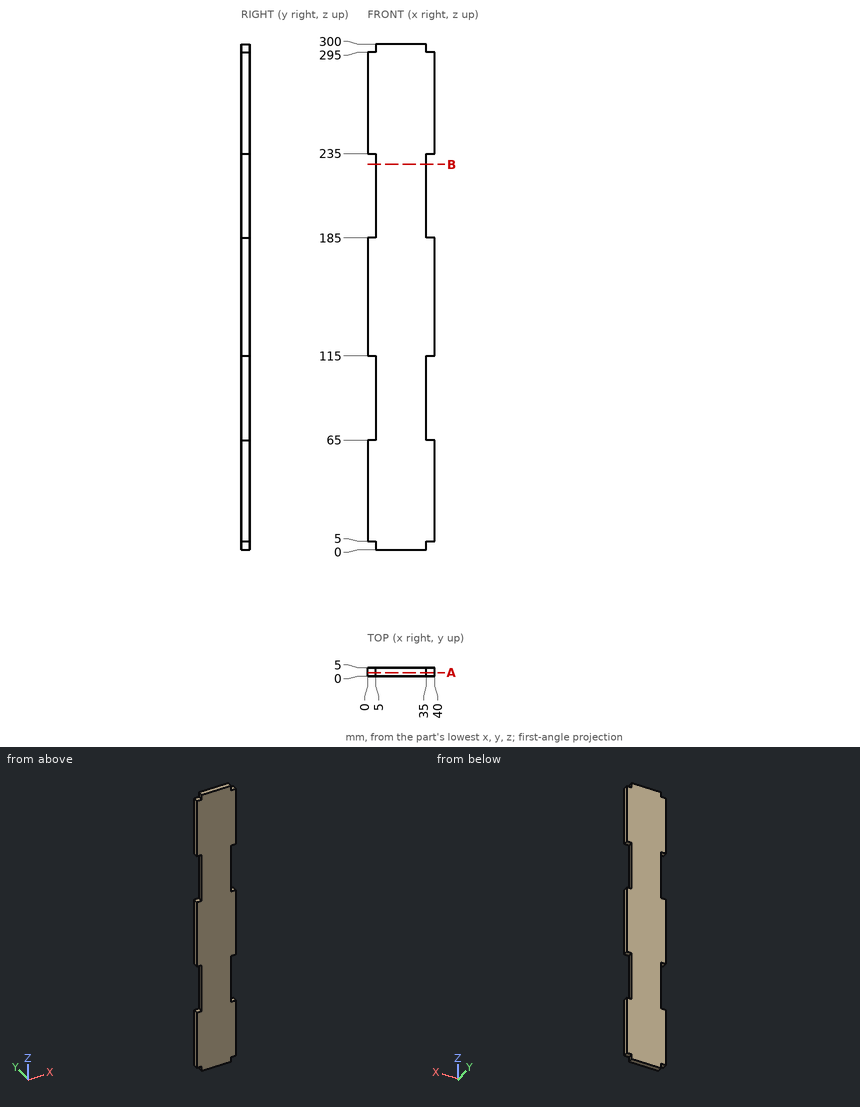
Answer from the drawing. Dimensions are ordinates in mm from the lowest x, y and z of the part. Round coordinates to 2 decimals unless told otherwise and drop trailing zeros. Order: outer loops, then holes, each group sorted by start corner. A loop starts at its lowest first (then second) coordinate and runs counter-clockwise, first axis right, second up.
1) The part is cut by section A-A on y = 2. Write down the section's boundary in (x, z).
2) Straight lines are drawn through the part: L1, parallel to Z at x = 3.5, y = 3.95; L2, parallel to X at y = 0.75, z = 208. For each, find the intervals that lie inside material, in ascending order.
3) Flat-ended cylindrical pins translate along their axes: pin 1 (1.5 mm diameter, centred on x = 36.5, y = 3.5, fed in from -Z); pin 2 (2.5 mm diameter, centred on y = 3, z = 296.5, fed in from +X); pin 3 (2.5 mm diameter, centred on y = 2.5, z = 216, fed in from -X); pin 4 (2 mm diameter, centred on x = 27.5, y = 4, fed in from -Z). Find the tip coordinate at first contact, or state that the pin passes through.
4) The part is cut by section B-B on z = 228.5. Write down the section's boundary in (x, y), plus the area to 3 significant figures.
Resolved:
1. outline: (0, 5) - (5, 5) - (5, 0) - (35, 0) - (35, 5) - (40, 5) - (40, 65) - (35, 65) - (35, 115) - (40, 115) - (40, 185) - (35, 185) - (35, 235) - (40, 235) - (40, 295) - (35, 295) - (35, 300) - (5, 300) - (5, 295) - (0, 295) - (0, 235) - (5, 235) - (5, 185) - (0, 185) - (0, 115) - (5, 115) - (5, 65) - (0, 65) - close
2. L1: z = 5 to 65, 115 to 185, 235 to 295
2. L2: x = 5 to 35
3. pin 1: stops at z = 5
3. pin 2: stops at x = 35
3. pin 3: stops at x = 5
3. pin 4: stops at z = 0
4. outline: (5, 0) - (35, 0) - (35, 5) - (5, 5) - close
4. area: 150 mm2
